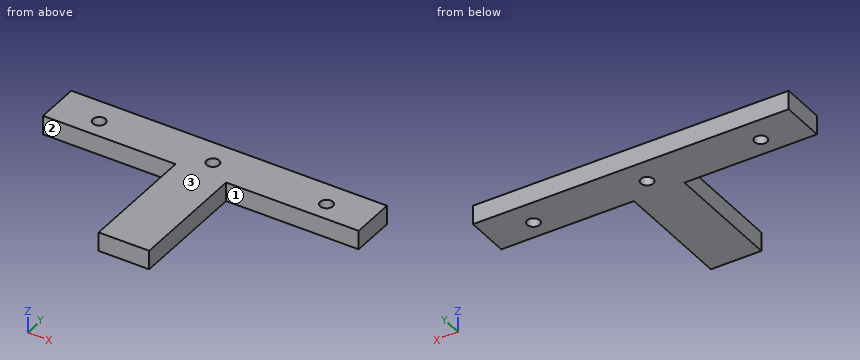
from build123d import *

# Parameters (mm, degrees)
EXTRUDE_1_DEPTH     = 15
SKETCH_2_R          = 5
CUT_EXTRUDE_1_DEPTH = 212.504412291


with BuildPart() as part:
    # 草圖1 → 填料-伸長1 (new body)
    with BuildSketch(Plane.XY):
        Polygon((-15.155141061, 7.219614063), (-55.155141061, 7.219614063), (-55.155141061, 102.329702578), (-160.155141061, 102.329702578), (-160.155141061, 137.329702578), (89.844858939, 137.329702578), (89.844858939, 102.329702578), (-15.155141061, 102.329702578), align=None)
    extrude(amount=EXTRUDE_1_DEPTH)

    # 草圖2 → 除料-伸長1 (cut, through all)
    with BuildSketch(Plane.XY.offset(15)):
        with Locations((54.844858939, 117.189491535)):
            Circle(SKETCH_2_R)
        with Locations((-35.155141061, 117.189491535)):
            Circle(SKETCH_2_R)
        with Locations((-125.155141061, 117.189491535)):
            Circle(SKETCH_2_R)
    extrude(amount=-CUT_EXTRUDE_1_DEPTH, mode=Mode.SUBTRACT)


solid = part.part
Read the model definition and answer for the solid it produces. Units are mm, in the model's axes. Face numbers are marked on the shaded views. A direction names the side the tool comes from. Coordinates: 2 decimals unless noted, no trailing zeros. Order: outer loops, then holes, each group sorted by start corner. A loop starts at its lowest first (then second) coordinate and runs counter-clockwise, first axis right, second up. Notation, with made-up numbers: (72.5, 52) -> (113.5, 52) arc R31 ccw to (113.5, 89) -> close; hole circle Ø8 at (50, -19.75). An arc over 180 degrees is marked (long way). Answer as a JSON object with one key per item and string values.
1) Consider line 1 along X through (y, z) = (89.5, 10.5); line 2 along Y through (x, z) = (-62, 9.5); line 3 along X through (y, z) = (113, 1.75). Determine where each line is inside the solid, lowest interval first. Write a range as from..to.
Model answer:
{"line 1": "x = -55.16..-15.16", "line 2": "y = 102.33..137.33", "line 3": "x = -160.16..-127.88, -122.43..-37.88, -32.43..52.12, 57.57..89.84"}
2) A cutting plane is placed at C-C, the plane x = -78. Determine the outline of the cut face in (y, z), plus the area to 3 significant figures.
Model answer:
{"outline": "(102.33, 0) -> (137.33, 0) -> (137.33, 15) -> (102.33, 15) -> close", "area": "525 mm²"}
3) A cutting plane is placed at B-B, the plane y = 89.5. Determine the outline of the cut face in (x, z).
Model answer:
{"outline": "(-55.16, 0) -> (-15.16, 0) -> (-15.16, 15) -> (-55.16, 15) -> close"}
4) Each of these flat-tipped pins is pushed along its axis until it touches: pin 1 (3 mm diameter, centred on y = 51, z = 3.5, fed in from -X); pin 2 (7.5 mm diameter, centred on x = -133.5, z = 9, fed in from -Y); pin 3 (1 mm diameter, centred on y = 29.5, z = 4, fed in from +X). Where does it stop, or does it pass through?
Model answer:
{"pin 1": "stops at x = -55.16", "pin 2": "stops at y = 102.33", "pin 3": "stops at x = -15.16"}
5) A tool of negligible diameter and unlimited length cuts with its end or side. For the marked faces 1, 2 and 3, from which of +Z, -Z, +X, -X, +Y, -Y can it reach the whole face along a straight path? Write none if from no direction.
Model answer:
{"face 1": "+Z, -Z, +X, -Y", "face 2": "+Z, -Z, -X, -Y", "face 3": "+Z, +X, -X, +Y, -Y"}
6) A cutting plane is placed at A-A, the plane z = 3.5. Determine the outline of the cut face in (x, y), plus the area to 3 significant figures.
Model answer:
{"outline": "(-160.16, 102.33) -> (-55.16, 102.33) -> (-55.16, 7.22) -> (-15.16, 7.22) -> (-15.16, 102.33) -> (89.84, 102.33) -> (89.84, 137.33) -> (-160.16, 137.33) -> close; hole circle Ø10 at (-125.16, 117.19); hole circle Ø10 at (-35.16, 117.19); hole circle Ø10 at (54.84, 117.19)", "area": "12,300 mm²"}
